Could you check a few things on this model? Use its own coordinates, in mm. Face numbers are marked on the shaded views. A direction names the side the tool comes from. Round coordinates to 2 decimals unless told otherwise and drop trailing zeros. Write each loop counter-clockwise with the first axis right and the second up, starting at its lowest first coordinate (ties: lowest second). Pieces come first, ordered by that corner, then holes. Notation, with made-up numbers: (48.5, 24) - (75.5, 24) arc R27 cw to (75.5, 57) - close; hole circle Ø4 at (76.25, 24). An arc over 180 degrees is marked (long way). Put each result on its own line as item: value.
from build123d import *

# Parameters (mm, degrees)
RESSALTO_EXTRUS_O1_DEPTH = 16
ESBO_O5_R                = 4.5
CORTE_EXTRUS_O1_DEPTH    = 51.695167423


with BuildPart() as part:
    # Esboço2 → Ressalto-extrusão1 (new body)
    with BuildSketch(Plane.XY):
        with BuildLine():
            Line((0, 33), (0, 0))
            Line((0, 0), (18, 0))
            Line((18, 0), (18, 16.5))
            ThreePointArc((18, 16.5), (16.939339828, 19.060660172), (19.5, 18))
            Line((19.5, 18), (35, 18))
            Line((35, 18), (35, 33))
            Line((35, 33), (0, 33))
        make_face()
    extrude(amount=RESSALTO_EXTRUS_O1_DEPTH)

    # Esboço5 → Corte-extrusão1 (cut, through all)
    with BuildSketch(Plane(origin=(35, 0, 0), x_dir=(0, 0, -1), z_dir=(1, 0, 0))):
        with Locations(Location((-8, 25.5, 0), (0, 0, 90))):
            Circle(ESBO_O5_R)
    extrude(amount=-CORTE_EXTRUS_O1_DEPTH, mode=Mode.SUBTRACT)


solid = part.part
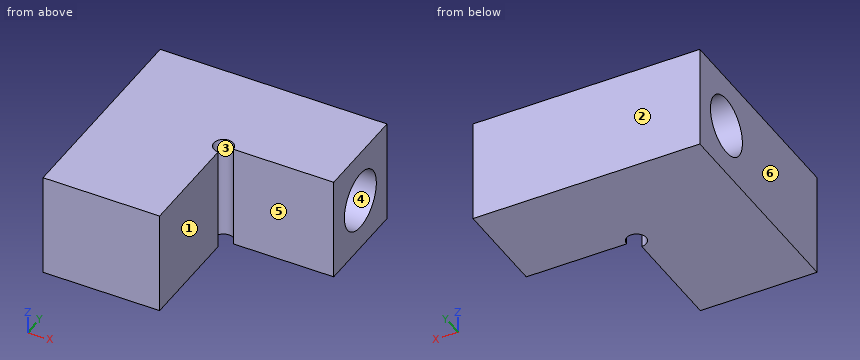
(1) Imagine slicing it at D-D, the plane x = 9. List the corners of the cut face in (y, z) for me, then the cut area to 3 significant figures.
Values found:
outline: (0, 0) - (33, 0) - (33, 16) - (0, 16) - close; hole circle Ø9 at (25.5, 8)
area: 464 mm^2
(2) For the marked faces 1 and 2, which set-ups out of +Z, -Z, +X, -X, +Y, -Y let a thin tool reach every point of the face, with its end or its side?
Values found:
face 1: +Z, -Z, +X, -Y
face 2: +Z, -Z, +X, -X, +Y
(3) Imagine slicing it at A-A, the plane y = 25.5. List the corners of the cut face in (x, z) for me.
Values found:
outline: (0, 0) - (35, 0) - (35, 3.5) - (0, 3.5) - close; (0, 12.5) - (35, 12.5) - (35, 16) - (0, 16) - close
(4) Imagine slicing it at B-B, the plane x = 17. List the corners of the cut face in (y, z) for me.
Values found:
outline: (0, 0) - (16.88, 0) - (16.88, 16) - (0, 16) - close; (19.12, 0) - (33, 0) - (33, 16) - (19.12, 16) - close; hole circle Ø9 at (25.5, 8)
(5) I'm going to push flat-ended pins straight in: pin 1 (6 mm diameter, centred on y = 14, z = 2.5, fed in from +X); pin 2 (8 mm diameter, centred on x = 28, z = 4, fed in from -Y); pin 3 (2.5 mm diameter, centred on x = 18, y = 18, fed in from +Z). Where does each tip first touch, or does it pass through?
Values found:
pin 1: stops at x = 18
pin 2: stops at y = 18
pin 3: passes through
(6) Imagine slicing it at C-C, the plane z = 6. List the corners of the cut face in (x, y) for me.
Values found:
outline: (0, 0) - (18, 0) - (18, 16.5) arc R1.5 cw (long way) to (19.5, 18) - (35, 18) - (35, 21.47) - (0, 21.47) - close; (0, 29.53) - (35, 29.53) - (35, 33) - (0, 33) - close
(7) Please list where these lines run through material, in increasing order: probe 1 along Z at (x, y) = (21, 25.5); probe 2 along X at (y, z) = (6.5, 2.25); probe 3 along Y at (x, z) = (10, 10.5). Write a range as from..to.
Values found:
probe 1: z = 0..3.5, 12.5..16
probe 2: x = 0..18
probe 3: y = 0..21.76, 29.24..33
(8) If we mould it in two halves opening along Y, with no side actions, what happens to the marked faces 3, 4, 5 and 6? For each: pulls with the +Y half, pulls with the -Y half, needs draft (parallel to the pull), parting line crosses it, or undercut.
Values found:
face 3: undercut
face 4: undercut
face 5: pulls with the -Y half
face 6: needs draft
